```python
from build123d import *

# Parameters (mm, degrees)
SKETCH_1_W          = 43
SKETCH_1_H          = 43
EXTRUDE_1_DEPTH     = 7.8
SKETCH_3_W          = 43
SKETCH_3_H          = 43
EXTRUDE_2_DEPTH     = 7.8
EXTRUDE_3_DEPTH     = 3.8
CUT_EXTRUDE_1_DEPTH = 47.5138689
SKETCH_6_W          = 10.365035434
SKETCH_6_H          = 2.8
EXTRUDE_5_DEPTH     = 2.8


with BuildPart() as part:
    # 草图1 → 凸台-拉伸1 (new body)
    with BuildSketch(Plane.XY):
        Rectangle(SKETCH_1_W, SKETCH_1_H)
    extrude(amount=EXTRUDE_1_DEPTH)

    # 草图3 → 凸台-拉伸2 (add)
    with BuildSketch(Plane.XZ.offset(21.5)):
        with Locations((0, 21.5)):
            Rectangle(SKETCH_3_W, SKETCH_3_H)
    extrude(amount=-EXTRUDE_2_DEPTH)

    # 草图4 → 凸台-拉伸3 (add)
    with BuildSketch(Plane.ZY.offset(21.5)):
        Polygon((7.8, 16.5), (38, -13.7), (7.8, -13.7), align=None)
    extrude_3 = extrude(amount=-EXTRUDE_3_DEPTH)

    # 镜向1: 凸台-拉伸3 across plane
    add(extrude_3.mirror(Plane(origin=(0, 0, 0), x_dir=(0, 0, 1), z_dir=(1, 0, 0))))

    # 草图5 → 切除-拉伸1 (cut, through all)
    with BuildSketch(Plane.XY.offset(7.8)):
        with BuildLine():
            Line((-4.25, 2.05), (-4.25, 6.3))
            Line((-4.25, 6.3), (-4.75, 6.3))
            ThreePointArc((-4.75, 6.3), (-9, 10.55), (-4.75, 14.8))
            Line((-4.75, 14.8), (4.75, 14.8))
            ThreePointArc((4.75, 14.8), (9, 10.55), (4.75, 6.3))
            Line((4.75, 6.3), (4.25, 6.3))
            Line((4.25, 6.3), (4.25, 2.05))
            ThreePointArc((4.25, 2.05), (0, -2.2), (-4.25, 2.05))
        make_face()
    cut_extrude_1 = extrude(amount=-CUT_EXTRUDE_1_DEPTH, mode=Mode.SUBTRACT)

    # 镜向2: 切除-拉伸1 across plane
    add(cut_extrude_1.mirror(Plane(origin=(0, -10.75, 10.75), x_dir=(0, 0.7071067811865478, 0.7071067811865472), z_dir=(0, 0.7071067811865475, -0.7071067811865477))), mode=Mode.SUBTRACT)

    # 草图6 → 凸台-拉伸5 (add)
    with BuildSketch(Plane.XZ.offset(21.5)):
        with Locations((0, 40.55829283)):
            Rectangle(SKETCH_6_W, SKETCH_6_H)
    extrude(amount=EXTRUDE_5_DEPTH)


solid = part.part
```
Here's how the part is built. I have some questions about the finished solid (model axes, mm). A direction names the side the tool comes from. Give positions to 0.01 mm unless a question says otherwise; leave off trailing zeros. Write each loop counter-clockwise with the first axis right and the second up, starting at its lowest first coordinate (ties: lowest second). Pieces come first, ordered by that corner, then holes.
(1) Imagine slicing it at A-A, the plane z = 24.5. Write out the boundary of the cut face in (x, y).
Output values:
outline: (-21.5, -21.5) - (-4.25, -21.5) - (-4.25, -13.7) - (-17.7, -13.7) - (-17.7, -0.2) - (-21.5, -0.2) - close; (4.25, -21.5) - (21.5, -21.5) - (21.5, -0.2) - (17.7, -0.2) - (17.7, -13.7) - (4.25, -13.7) - close
(2) Will these pins go through, and if not, where does the flat tip stop? pin 1 (3 mm diameter, centred on x = 8.5, y = 0, fed in from -Z); pin 2 (2 mm diameter, centred on y = -23, z = 41, fed in from +X); pin 3 (10.5 mm diameter, centred on x = 1, y = 1, fed in from +Z); pin 4 (1.4 mm diameter, centred on x = -1.5, y = -22.5, fed in from -Z).
Output values:
pin 1: stops at z = 0
pin 2: stops at x = 5.18
pin 3: stops at z = 7.8
pin 4: stops at z = 39.16
(3) Imagine slicing it at B-B, the plane x = 0. Write out the boundary of the cut face in (y, z).
Output values:
outline: (-24.3, 39.16) - (-21.5, 39.16) - (-21.5, 36.3) - (-13.7, 36.3) - (-13.7, 43) - (-21.5, 43) - (-21.5, 41.96) - (-24.3, 41.96) - close; (-21.5, 0) - (-2.2, 0) - (-2.2, 7.8) - (-13.7, 7.8) - (-13.7, 19.3) - (-21.5, 19.3) - close; (14.8, 0) - (21.5, 0) - (21.5, 7.8) - (14.8, 7.8) - close
(4) On a 3-axis mill with a long thin cutter (end or side, diameter ignored), from which of +Z, -Z, +X, -X, +Y, -Y can I reach the whole of each face in a straight line? I mean faces 5 (the face through (0, -23, 41.958)), 6 (the face through (0, 14.8, 4)), 7 (the face through (-5, -13.7, 26)), 8 (the face through (9, -18, 32)). Say none if no direction works.
Output values:
face 5: +Z, +X, -X, -Y
face 6: +Z, -Z
face 7: +Z, +Y
face 8: +Y, -Y
(5) If I drill on L1, parallel to X at y = 3, z = 15; L2, parallel to Y at x = -4, z = 16; L3, parallel to Z at x = -6.5, y = -6, over which ranges is the centre line in solid material (lowest first)?
Output values:
L1: x = -21.5 to -17.7, 17.7 to 21.5
L2: y = -21.5 to -13.7
L3: z = 0 to 7.8
(6) Thinking about a two-plate mould opening in X: for faces 1 (the face through (0.1, -17.5, 19.3)), 2 (the face through (-5.183, -23, 41)), 3 (the face through (-4.25, -18, 26)), 4 (the face through (-19.6, 1.6, 22.7)), which applies, pulls with the +X half, pulls with the -X half, needs draft (parallel to the pull), parting line crosses it, or undercut?
Output values:
face 1: undercut
face 2: pulls with the -X half
face 3: undercut
face 4: needs draft
(7) Imagine slicing it at C-C, the plane y = 3.5. Write out the boundary of the cut face in (x, z).
Output values:
outline: (-21.5, 0) - (-4.25, 0) - (-4.25, 7.8) - (-17.7, 7.8) - (-17.7, 20.8) - (-21.5, 20.8) - close; (4.25, 0) - (21.5, 0) - (21.5, 20.8) - (17.7, 20.8) - (17.7, 7.8) - (4.25, 7.8) - close
(8) Imagine slicing it at D-D, the plane y = -3.5. Write out the boundary of the cut face in (x, z), and give its area (3 significant figures).
Output values:
outline: (-21.5, 0) - (21.5, 0) - (21.5, 27.8) - (17.7, 27.8) - (17.7, 7.8) - (-17.7, 7.8) - (-17.7, 27.8) - (-21.5, 27.8) - close
area: 487 mm2
